```python
from build123d import *

# Parameters (mm, degrees)
DODANIE_WYCI_GNI_CIE1_DEPTH = 12.5
SKORUPA2_START              = -10.714285714
SKORUPA2_OUTLINE_W          = 37
SKORUPA2_OUTLINE_H          = 21
SKORUPA2_DEPTH              = 23
SZKIC2_R                    = 3
SZKIC2_R_2                  = 4
WYTNIJ_WYCI_GNI_CIE1_DEPTH  = 60


# Read off the part's stored shape, not the designer's step: Skorupa2
with BuildPart() as part:
    # Szkic1 → Dodanie-wyciągnięcie1 (new, symmetric)
    with BuildSketch(Plane.XY):
        with BuildLine():
            Line((20, 12.285714286), (-3, -10.714285714))
            Line((-3, -10.714285714), (-15, -10.714285714))
            ThreePointArc((-15, -10.714285714), (-2.5, 1.785714286), (-15, 14.285714286))
            Line((-15, 14.285714286), (20, 14.285714286))
            Line((20, 14.285714286), (20, 12.285714286))
        make_face()
    extrude(amount=DODANIE_WYCI_GNI_CIE1_DEPTH, both=True)

    # Skorupa2 outline → Skorupa2 (cut)
    with BuildSketch(Plane(origin=(0, 0, 0), x_dir=(1, 0, 0), z_dir=(0, 1, 0)).offset(SKORUPA2_START)):
        with Locations((2.5, 0)):
            Rectangle(SKORUPA2_OUTLINE_W, SKORUPA2_OUTLINE_H)
    extrude(amount=SKORUPA2_DEPTH, mode=Mode.SUBTRACT)

    # Szkic2 → Wytnij-wyciągnięcie1 (cut)
    with BuildSketch(Plane(origin=(0, 14.285714286, 0), x_dir=(1, 0, 0), z_dir=(0, 1, 0))):
        with Locations(Location((10, 0, 0), (0, 0, 180))):
            Circle(SZKIC2_R)
        with Locations((8, -24.919871589)):
            Circle(SZKIC2_R_2)
    extrude(amount=-WYTNIJ_WYCI_GNI_CIE1_DEPTH, mode=Mode.SUBTRACT)


solid = part.part
```
Model file for the job. Use its own axes, mm. A direction names the side the tool comes from. Coordinates: 2 decimals unless noted, no trailing zeros. Loops run counter-clockwise (first coordinate to the right, second up) from the corner with the lowest first, then second, coordinate; pieces in that order, holes last. Notation, with made-up numbers: (85, 86.25) -> (91, 86.25) arc R19 cw to (91, 101.25) -> close; hole circle Ø8 at (-35.75, -17). An arc over 180 degrees is marked (long way). Answer as a JSON object with one key per item and string values.
Q1. Cut at D-D (x = 14). List the corners of the cut face in (y, z), and give its area (3 significant figures).
Report:
{"outline": "(6.29, -12.5) -> (14.29, -12.5) -> (14.29, 12.5) -> (6.29, 12.5) -> (6.29, 10.5) -> (12.29, 10.5) -> (12.29, -10.5) -> (6.29, -10.5) -> close", "area": "74.0 mm2"}
Q2. Cut at B-B (y = 5.5). List the corners of the cut face in (x, z).
Report:
{"outline": "(-3.06, -12.5) -> (13.21, -12.5) -> (13.21, -10.5) -> (-3.06, -10.5) -> close; (-3.06, 10.5) -> (13.21, 10.5) -> (13.21, 12.5) -> (-3.06, 12.5) -> close"}
Q3. Flat gauge pin, fed straight in: P1, Ø10, axis at x = -5, z = 3, coming from the -Y side. Where does the tip first touch, or does it go through?
Report:
{"P1": "stops at y = 12.29"}
Q4. Pull direction X, two halves, no side cores. Call faces 3 (the cylindrical face through (13, 13, 0)), 4 (the flat face through (2, 14.286, 0)), 5 (the cylindrical face through (-8.51, 12.47, 0.18)): released by +X, released by -X, zero draft, split by the parting line, or undercut.
Report:
{"face 3": "undercut", "face 4": "zero draft", "face 5": "released by -X"}
Q5. Cut at C-C (x = 10). List the corners of the cut face in (y, z), and give its area (3 significant figures).
Report:
{"outline": "(2.29, -12.5) -> (14.29, -12.5) -> (14.29, -3) -> (12.29, -3) -> (12.29, -10.5) -> (2.29, -10.5) -> close; (2.29, 10.5) -> (12.29, 10.5) -> (12.29, 3) -> (14.29, 3) -> (14.29, 12.5) -> (2.29, 12.5) -> close", "area": "78.0 mm2"}
Q6. 3-axis set-ups, long thin cutter, end or side, ignore diameter. For faces 1 (the flat face through (-9, -10.714, -11)), 2 (the flat face through (2, 3, 10.5)): which of +Z, -Z, +X, -X, +Y, -Y reach the whole face in a straight line?
Report:
{"face 1": "+Z, -Z, +X, -X, -Y", "face 2": "+X, -X, -Y"}
Q7. Cut at A-A (z = 0). List the corners of the cut face in (x, y), and give its area (3 significant figures).
Report:
{"outline": "(-15, 14.29) arc R12.5 cw to (-8.22, 12.29) -> (7, 12.29) -> (7, 14.29) -> close; (13, 12.29) -> (20, 12.29) -> (20, 14.29) -> (13, 14.29) -> close", "area": "48.8 mm2"}
Q8. Probe probe 1 along Z at (x, y) = (10, 13.5); probe 2 along Z at (x, y) = (3, 2.5); probe 3 along Y at (x, z) = (14, -2.75). List the from-to ranges inside material, lowest first.
Report:
{"probe 1": "z = -12.5 to -3, 3 to 12.5", "probe 2": "z = -12.5 to -10.5, 10.5 to 12.5", "probe 3": "y = 12.29 to 14.29"}
